from build123d import *

# Parameters (mm, degrees)
SKETCH1_W            = 127
SKETCH1_H            = 40.64
BOSS_EXTRUDE1_DEPTH  = 5.08
CHAMFER3_SIZE        = 2.54
SKETCH6_W            = 127
SKETCH6_H            = 19.05
BOSS_EXTRUDE4_DEPTH  = 12.7
SKETCH14_R           = 3.175
BOSS_EXTRUDE9_DEPTH  = 19.05
SKETCH15_R           = 9.525
BOSS_EXTRUDE10_DEPTH = 5.08
SKETCH16_W           = 28.22730188
SKETCH16_H           = 7.62
BOSS_EXTRUDE11_DEPTH = 5.08
SKETCH17_W           = 26.13431135
SKETCH17_H           = 5.08
CUT_EXTRUDE4_DEPTH   = 5.08
SKETCH18_W           = 127
SKETCH18_H           = 0.254
BOSS_EXTRUDE12_DEPTH = 0.254


with BuildPart() as part:
    # Sketch1 → Boss-Extrude1 (new body)
    with BuildSketch(Plane.XY):
        with Locations((63.5, 20.32)):
            Rectangle(SKETCH1_W, SKETCH1_H)
    extrude(amount=BOSS_EXTRUDE1_DEPTH)

    # Chamfer3
    chamfer3_edges = [part.edges().sort_by_distance(p)[0] for p in [
        (63.5, 0, 5.08),
    ]]
    chamfer(chamfer3_edges, length=CHAMFER3_SIZE)

    # Sketch6 → Boss-Extrude4 (add)
    with BuildSketch(Plane.XY.offset(5.08)):
        with Locations((63.5, 31.115)):
            Rectangle(SKETCH6_W, SKETCH6_H)
    extrude(amount=BOSS_EXTRUDE4_DEPTH)

    # Sketch14 → Boss-Extrude9 (add)
    with BuildSketch(Plane.XY.offset(17.78)):
        with Locations((25.4, 29.21)):
            Circle(SKETCH14_R)
    extrude(amount=BOSS_EXTRUDE9_DEPTH)

    # Sketch15 → Boss-Extrude10 (add)
    with BuildSketch(Plane.XY.offset(36.83)):
        with Locations((25.4, 29.21)):
            Circle(SKETCH15_R)
    extrude(amount=BOSS_EXTRUDE10_DEPTH)

    # Sketch16 → Boss-Extrude11 (add)
    with BuildSketch(Plane.XY.offset(17.78)):
        with Locations((26.81365094, 36.83)):
            Rectangle(SKETCH16_W, SKETCH16_H)
    extrude(amount=BOSS_EXTRUDE11_DEPTH)

    # Sketch17 → Cut-Extrude4 (cut)
    with BuildSketch(Plane.XY.offset(22.86)):
        with Locations((26.783155675, 36.83)):
            Rectangle(SKETCH17_W, SKETCH17_H)
    extrude(amount=-CUT_EXTRUDE4_DEPTH, mode=Mode.SUBTRACT)

    # Sketch18 → Boss-Extrude12 (add)
    with BuildSketch(Plane(origin=(0, 0, 0), x_dir=(-1, 0, 0), z_dir=(0, 0, -1))):
        with Locations((-63.5, 27.813)):
            Rectangle(SKETCH18_W, SKETCH18_H)
    extrude(amount=BOSS_EXTRUDE12_DEPTH)


solid = part.part
Here's how the part is built. I have some questions about the finished solid (model axes, mm). A direction names the side the tool comes from. Round coordinates to 2 decimals unless told otherwise and drop trailing zeros. Write each loop counter-clockwise with the first axis right and the second up, starting at its lowest first coordinate (ties: lowest second). Pieces come first, ordered by that corner, then holes.
1. If we mould it in two halves opening along Y, with no side actions, what happens to faces 1 (the flat face through (39.85, 37, 20)), 2 (the flat face through (27, 39.37, 20)), 3 (the flat face through (63, 34, 0)), 4 (the cylindrical face through (15.884, 29.629, 39.334))? For each: released by +Y, released by -Y, zero draft, split by the parting line, or undercut.
2. For faces 5 (the cylindrical face through (28.33, 27.99, 27.17)), 6 (the flat face through (40.927, 37, 20)), 7 (the flat face through (12.7, 37, 20)), which set-ups out of +Z, -Z, +X, -X, +Y, -Y let a thin tool reach every point of the face, with its end or its side?
3. Suppose I cut it at C-C (x = 79). List the corners of the cut face in (y, z) for me.
4. Suppose I cut it at A-A (x = 31.5). List the corners of the cut face in (y, z) for me.
5. I need wall thicknesses on L1, parallel to Z at x = 29.5, y = 31; L2, parallel to Y at x = 72, z = 8.5; L3, parallel to Z at x = 105, y = 7. Which ranges of each line are inside material? Lowest first, please.
6. Will these pins go through, and if not, where does the flat tip stop? pin 1 Ø1 at (y, z) = (27.5, 19) entering from -X; pin 2 Ø4 at (y, z) = (36.5, 21.5) entering from +X; pin 3 Ø12 at (x, z) = (16, 33.5) entering from +Y.
7. Suppose I cut it at B-B (y = 29.21). List the corners of the cut face in (x, z) for me (3 decimals), and give its area (3 significant figures).
8. Suppose I cut it at D-D (z = 29.5). List the corners of the cut face in (x, y) for me (3 decimals), and give its area (3 significant figures).
Answer sheet:
1. face 1: undercut
1. face 2: undercut
1. face 3: zero draft
1. face 4: split by the parting line
2. face 5: none
2. face 6: +Z, +X, +Y, -Y
2. face 7: +Z, -X, +Y, -Y
3. outline: (0, 0) - (27.69, 0) - (27.69, -0.25) - (27.94, -0.25) - (27.94, 0) - (40.64, 0) - (40.64, 17.78) - (21.59, 17.78) - (21.59, 5.08) - (2.54, 5.08) - (0, 2.54) - close
4. outline: (0, 0) - (27.69, 0) - (27.69, -0.25) - (27.94, -0.25) - (27.94, 0) - (40.64, 0) - (40.64, 22.86) - (39.37, 22.86) - (39.37, 17.78) - (34.29, 17.78) - (34.29, 22.86) - (33.02, 22.86) - (33.02, 17.78) - (21.59, 17.78) - (21.59, 5.08) - (2.54, 5.08) - (0, 2.54) - close; (21.89, 36.83) - (36.53, 36.83) - (36.53, 41.91) - (21.89, 41.91) - close
5. L1: z = 0 to 17.78, 36.83 to 41.91
5. L2: y = 21.59 to 40.64
5. L3: z = 0 to 5.08
6. pin 1: stops at x = 22.46
6. pin 2: stops at x = 40.93
6. pin 3: stops at y = 37.65
7. outline: (0, 0) - (127, 0) - (127, 17.78) - (28.575, 17.78) - (28.575, 36.83) - (34.925, 36.83) - (34.925, 41.91) - (15.875, 41.91) - (15.875, 36.83) - (22.225, 36.83) - (22.225, 17.78) - (0, 17.78) - close
7. area: 2,480 mm2
8. outline: circle Ø6.35 at (25.4, 29.21)
8. area: 31.7 mm2
